Here's how the part is built. I have some questions about the finished solid (model axes, mm). Face numbers are marked on the shaded views. A direction names the side the tool comes from. Round coordinates to 2 decimals unless told otherwise and drop trailing zeros. Loops run counter-clockwise (first coordinate to the right, second up) from the corner with the lowest first, then second, coordinate; pieces in that order, holes last. Notation, with made-up numbers: (8, 33.5) - (22, 33.5) arc R14 cw to (22, 38.5) - close; hole circle Ø5 at (-10.5, 54.5). An arc over 180 degrees is marked (long way). Answer as a JSON object with one key per item and string values. Group by question number.
1) Will these pins go through, and if not, where does the flat tip stop? P1, Ø4, axis at x = 41, y = 5, coming from the +Z side; P2, Ø3, axis at y = 18, z = 9, coming from the +X side; P3, Ø3.5, axis at x = 56, z = 3, coming from the -Y side.
2) I want a section at D-D, the plane y = 5. Please give me the cut outline in (x, z).
3) If I drill on line 1 along X through (y, z) = (34.5, 3.5); line 2 along Y through (x, z) = (10, 2); line 3 along X through (y, z) = (32, 8.5), over which ranges is the centre line in solid material (lowest first)? Write a range as [from, to].
4) If we mould it in two halves opening along Y, with no side actions, what happens to the marked faces 1, 2 and 3? For each: pulls with the +Y half, pulls with the -Y half, needs draft (parallel to the pull), parting line crosses it, or undercut.
5) I want a section at A-A, the plane y = 50. Please give me the cut outline in (x, z), then the cut area to 3 significant figures.
6) Which directions (+Z, -Z, +X, -X, +Y, -Y) give clear straight access to the entire face, cutting with the end or side of a thin tool? Please do the marked faces 4, 5, 6, 7 and 8.
7) I want a section at B-B, the plane x = 55. Please give me the cut outline in (y, z).
8) I want a section at C-C, the plane z = 4.75. Please give me the cut outline in (x, y), then the cut area to 3 significant figures.
from build123d import *

# Parameters (mm, degrees)
F0_R     = 2.75
F0_R_2   = 13.25
F1_DEPTH = 12
F2_R     = 4.25
F3_DEPTH = 6
F4_R     = 4.25
F5_DEPTH = 6


with BuildPart() as f1:
    # F0 (on Top) → F1 (new body)
    with BuildSketch(Plane.XY):
        Polygon((0, 38), (0, 0), (50, 0), (50, 30), (63, 30), (63, 58), (25, 58), align=None)
        with Locations((10, 5)):
            Circle(F0_R, mode=Mode.SUBTRACT)
        with Locations((25, 20)):
            Circle(F0_R_2, mode=Mode.SUBTRACT)
        with Locations((40, 5)):
            Circle(F0_R, mode=Mode.SUBTRACT)
        with Locations((10, 35)):
            Circle(F0_R, mode=Mode.SUBTRACT)
        with Locations((40, 35)):
            Circle(F0_R, mode=Mode.SUBTRACT)
        with Locations((55, 50)):
            Circle(F0_R, mode=Mode.SUBTRACT)
    extrude(amount=F1_DEPTH)

    # F2 (on face) → F3 (cut)
    with BuildSketch(Plane.XY.offset(12)):
        with Locations((10, 35)):
            Circle(F2_R)
        with Locations((40, 35)):
            Circle(F2_R)
        with Locations((10, 5)):
            Circle(F2_R)
        with Locations((40, 5)):
            Circle(F2_R)
    extrude(amount=-F3_DEPTH, mode=Mode.SUBTRACT)

    # F4 (on face) → F5 (cut)
    with BuildSketch(Plane(origin=(0, 0, 0), x_dir=(1, 0, 0), z_dir=(0, 0, -1))):
        with Locations((55, -50)):
            Circle(F4_R)
    extrude(amount=-F5_DEPTH, mode=Mode.SUBTRACT)


solid = f1.part
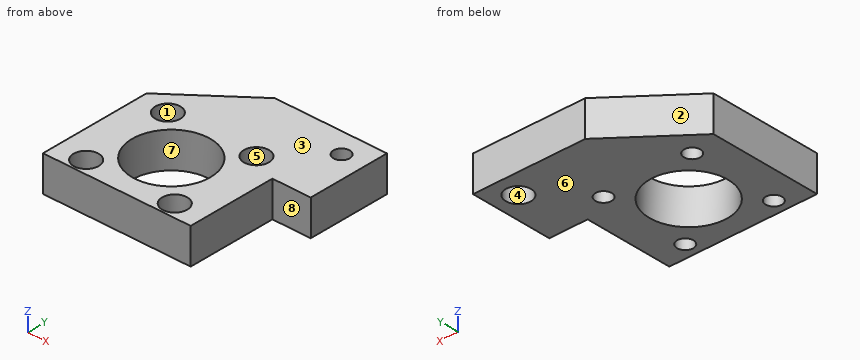
Outcome:
{
 "1": {"P1": "z = 6", "P2": "x = 50", "P3": "y = 30"},
 "2": {"outline": "(0, 0) - (7.25, 0) - (7.25, 6) - (5.75, 6) - (5.75, 12) - (0, 12) - close; (12.75, 0) - (37.25, 0) - (37.25, 6) - (35.75, 6) - (35.75, 12) - (14.25, 12) - (14.25, 6) - (12.75, 6) - close; (42.75, 0) - (50, 0) - (50, 12) - (44.25, 12) - (44.25, 6) - (42.75, 6) - close"},
 "3": {"line 1": "[0, 7.3], [12.7, 37.3], [42.7, 63]", "line 2": "[0, 2.25], [7.75, 32.25], [37.75, 46]", "line 3": "[0, 6.99], [13.01, 19.38], [30.62, 36.99], [43.01, 63]"},
 "4": {"face 1": "undercut", "face 2": "pulls with the +Y half", "face 3": "needs draft"},
 "5": {"outline": "(15, 0) - (50.75, 0) - (50.75, 6) - (52.25, 6) - (52.25, 12) - (15, 12) - close; (57.75, 6) - (59.25, 6) - (59.25, 0) - (63, 0) - (63, 12) - (57.75, 12) - close", "area": "492 mm^2"},
 "6": {"face 4": "-Z", "face 5": "+Z", "face 6": "-Z, +X, -X, +Y, -Y", "face 7": "+Z, -Z", "face 8": "+Z, -Z, +X, -Y"},
 "7": {"outline": "(30, 0) - (45.75, 0) - (45.75, 6) - (47.25, 6) - (47.25, 12) - (30, 12) - close; (52.75, 6) - (54.25, 6) - (54.25, 0) - (58, 0) - (58, 12) - (52.75, 12) - close"},
 "8": {"outline": "(0, 0) - (50, 0) - (50, 30) - (63, 30) - (63, 58) - (25, 58) - (0, 38) - close; hole circle Ø5.5 at (10, 5); hole circle Ø5.5 at (10, 35); hole circle Ø26.5 at (25, 20); hole circle Ø5.5 at (40, 5); hole circle Ø5.5 at (40, 35); hole circle Ø8.5 at (55, 50)", "area": "2,310 mm^2"}
}
